Design review of the part built by this model. Coordinates are the model's own, in mm. Face numbers are marked on the shaded views. A direction names the side the tool comes from. Coordinates: 2 decimals unless noted, no trailing zeros. Write each loop counter-clockwise with the first axis right and the second up, starting at its lowest first coordinate (ties: lowest second). Pieces come first, ordered by that corner, then holes. Notation, with made-up numbers: M 54.5,-8 L 72.5,-8 A12 ccw 72.5,8 Z; hole C 8.25,44 d7. An arc over 180 degrees is marked long. One line per question, with ' | ' between items.
Solid Edge part; units mm, degrees
sketch "Sketch1" plane through (0, 11, 0) normal (0, -1, 0) x (1, 0, 0)
  circle A0 centre (-10.5, -25) radius 2.2
  circle A1 centre (10.5, -25) radius 2.2
  line L0 (-38, 0) -> (-29, 0)
  line L1 (-29, 0) -> (-29, -4)
  line L2 (-21, -4) -> (-21, 0)
  line L3 (-21, 0) -> (-8, 0)
  line L4 (-8, 0) -> (-5, 0)
  line L5 (-5, 0) -> (-5, 2.6)
  line L6 (-5, 2.6) -> (5, 2.6)
  line L7 (5, 2.6) -> (5, 0)
  line L8 (8, 0) -> (5, 0)
  line L9 (21, 0) -> (8, 0)
  line L10 (21, -4) -> (21, 0)
  arc A2 (21, -4) -> (29, -4) centre (25, -4) ccw
  line L11 (29, 0) -> (29, -4)
  line L12 (38, 0) -> (29, 0)
  line L13 (38, 0) -> (38, -13)
  line L14 (38, -13) -> (28, -13)
  line L15 (28, -13) -> (16, -26)
  line L16 (16, -26) -> (16, -36)
  line L17 (16, -36) -> (5, -36)
  line L18 (5, -8) -> (5, -36)
  line L19 (0, -8) -> (5, -8)
  line L20 (0, -8) -> (-5, -8)
  line L21 (-5, -8) -> (-5, -36)
  line L22 (-16, -36) -> (-5, -36)
  line L23 (-16, -26) -> (-16, -36)
  line L24 (-28, -13) -> (-16, -26)
  line L25 (-38, -13) -> (-28, -13)
  line L26 (-38, 0) -> (-38, -13)
  arc A3 (-29, -4) -> (-21, -4) centre (-25, -4) ccw
  dimension "D1" = 38
  dimension "D2" = 38
  dimension "D3" = 38
  dimension "D4" = 38
extrude "ExtrudedProtrusion_1" add sketch "Sketch1" against normal blind 12
sketch "Sketch2" plane through (0, 17, -8) normal (0, 0, -1) x (1, 0, 0)
  circle A0 centre (0, 0) radius 2.2
extrude "Cutout1" cut sketch "Sketch2" against normal through all
sketch "Sketch3" plane through (33, 17, -13) normal (0, 0, -1) x (-1, 0, 0)
  circle A0 centre (-0.5, 0) radius 2.2
extrude "Cutout2" cut sketch "Sketch3" against normal through all
mirror "Mirror1" about plane through (0, 0, 0) normal (1, 0, 0) of "Cutout2"
sketch "Sketch4" plane through (16, 17, -31) normal (1, 0, 0) x (0, -1, 0)
  circle A0 centre (0, -0.5) radius 2.2
extrude "Cutout4" cut sketch "Sketch4" against normal through all
sketch "Sketch5" plane through (0, 23, -17.75) normal (0, 1, 0) x (0, 0, 1)
  line L0 (4.75, 16) -> (-17.25, 16)
  line L1 (4.75, 38) -> (4.75, 16)
extrude "Cutout5" cut sketch "Sketch5" against normal through all material side at (16.05, 23, -24)
sketch "Sketch6" plane through (0, 23, -16.75) normal (0, 1, 0) x (1, 0, 0)
  circle A0 centre (5, -4.75) radius 4
  circle A1 centre (16, -3.75) radius 4
extrude "Cutout6" cut sketch "Sketch6" against normal through all
sketch "Sketch7" plane through (0, 17, 2.6) normal (0, 0, 1) x (1, 0, 0)
  line L0 (0, 0) -> (1.5825, 1.5282)
  line L1 (1.5825, 1.5282) -> (0, 3.167)
  line L2 (0, 3.167) -> (-1.5825, 1.5282)
  line L3 (-1.5825, 1.5282) -> (0, 0)
  line L4 (33.5, 0) -> (35.0825, 1.5282)
  line L5 (35.0825, 1.5282) -> (33.5, 3.167)
  line L6 (33.5, 3.167) -> (31.9175, 1.5282)
  line L7 (31.9175, 1.5282) -> (33.5, 0)
  line L8 (-33.5, 0) -> (-31.9175, 1.5282)
  line L9 (-31.9175, 1.5282) -> (-33.5, 3.167)
  line L10 (-33.5, 3.167) -> (-35.0825, 1.5282)
  line L11 (-35.0825, 1.5282) -> (-33.5, 0)
extrude "Cutout7" cut sketch "Sketch7" against normal through all
sketch "Sketch8" plane through (-16, 17, -31) normal (-1, 0, 0) x (0, 0, 1)
  line L0 (0.5, 0) -> (2.0825, 1.5282)
  line L1 (2.0825, 1.5282) -> (0.5, 3.167)
  line L2 (0.5, 3.167) -> (-1.0825, 1.5282)
  line L3 (-1.0825, 1.5282) -> (0.5, 0)
extrude "Cutout8" cut sketch "Sketch8" against normal through all
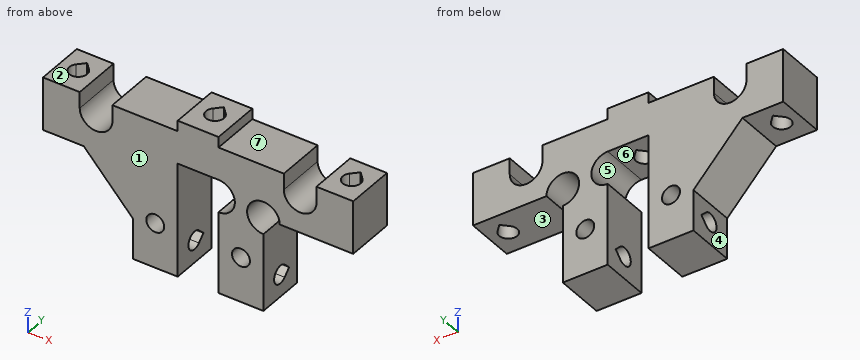
1. To check wall thickness, follow line 1 along X through (y, z) = (17, -0.25); line 2 along X through (y, z) = (20, -29.5); line 3 along X through (y, z) = (17, -24). State the ranges of each line that lie inside material, in increasing order. Write a range as [from, to].
Answer sheet:
line 1: [-38, -35.7], [-31.3, -29], [-21, -2.2], [2.2, 21], [29, 31.3], [35.7, 38] | line 2: [-16, -5], [5, 16] | line 3: [-17.85, -12.46], [-8.54, -5], [5, 8.54], [12.46, 16]
2. Take a section at B-B (z = -3). Write out the cut boundary in (x, y).
Answer sheet:
outline: M -38,11 L -29,11 L -29,23 L -38,23 Z; M -21,11 L 21,11 L 21,23 L -21,23 Z; M 29,11 L 38,11 L 38,23 L 29,23 Z; hole M -35.07,18.54 A2.2 ccw long -31.93,18.54 L -33.5,20.17 Z; hole M -1.57,18.54 A2.2 ccw long 1.57,18.54 L 0,20.17 Z; hole M 31.93,18.54 A2.2 ccw long 35.07,18.54 L 33.5,20.17 Z
3. Take a section at C-C (y = 17). Count the separate pieces of the cut face and the enclosed holes in it, then the cut area to 3 significant figures.
Answer sheet:
separate pieces: 6 | enclosed holes: 2 | area: 1,080 mm^2
4. Draft analysis for pull direction Y (two halves, no side actions). For the marked faces 1 and 2, state which applies: pulls with the +Y half, pulls with the -Y half, needs draft (parallel to the pull), parting line crosses it, or undercut.
Answer sheet:
face 1: pulls with the -Y half | face 2: needs draft
5. Insertion check: pin 1 Ø5.5 at (x, y) = (-33.5, 17) entering from -Z; pin 2 Ø7 at (x, y) = (0, 17) entering from -Z; pin 3 Ø3 at (y, z) = (13.5, -24) entering from -X; pin 4 Ø2.5 at (x, z) = (-10.5, -25) entering from -Y. Each pin has a flat end and moves straight along its axis. Give the tip position at first contact, or say it passes through.
Answer sheet:
pin 1: z = -13 | pin 2: z = -8 | pin 3: x = -19.23 | pin 4: through
6. Take a section at A-A (x = -10.5). Write out the cut boundary in (y, z), then the cut area to 3 significant figures.
Answer sheet:
outline: M 11,-36 L 23,-36 L 23,-27.2 L 11,-27.2 Z; M 11,-22.8 L 23,-22.8 L 23,0 L 11,0 Z; hole M 18.54,-32.07 L 20.17,-30.5 L 18.54,-28.93 A2.2 ccw long Z | area: 363 mm^2
7. Tool access review of the marked faces 3, 4, 5, 6 and 7: name each direction out of +Z, -Z, +X, -X, +Y, -Y from which nothing blocks a thin tool from reaching the whole face with its end or side.
Answer sheet:
face 3: -Z, +X, +Y, -Y | face 4: -Z, -X, +Y, -Y | face 5: +Y, -Y | face 6: -Z, +Y, -Y | face 7: +Z, +X, +Y, -Y
